from build123d import *

# Parameters (mm, degrees)
F1_DEPTH = 63.5
F2_DEPTH = 25.4
F3_DEPTH = 7.9375
F5_R     = 6.35


with BuildPart() as f1:
    # F0 (on Front) → F1 (new body, symmetric)
    with BuildSketch(Plane.XZ):
        Polygon((-41.275, 9.525), (-41.275, -9.525), (41.275, -9.525), (41.275, 9.525), (23.3043469489, 9.525), align=None)
    extrude(amount=F1_DEPTH, both=True)

    # F0 (on Front) → F2 (join, symmetric)
    with BuildSketch(Plane.XZ):
        with BuildLine():
            Line((23.3043469489, 9.525), (41.275, 9.525))
            Line((41.275, 9.525), (41.275, 32.9785965501))
            ThreePointArc((41.275, 32.9785965501), (47.109768429, 45.2753186743), (60.325, 48.5328564168))
            Line((60.325, 48.5328564168), (60.325, 66.675))
            ThreePointArc((60.325, 66.675), (34.3676792005, 58.0084605019), (23.3043469489, 32.9785965501))
            Line((23.3043469489, 32.9785965501), (23.3043469489, 9.525))
        make_face()
        with BuildLine():
            ThreePointArc((76.3579214275, 60.8458530511), (68.7147538428, 64.787159847), (60.325, 66.675))
            Line((60.325, 66.675), (60.325, 48.5328564168))
            ThreePointArc((60.325, 48.5328564168), (65.4413001724, 46.5163203784), (69.5626091196, 42.8752))
            Line((69.5626091196, 42.8752), (89.6713504766, 42.8752))
            Line((89.6713504766, 42.8752), (89.6713504766, 60.8458530511))
            Line((89.6713504766, 60.8458530511), (76.3579214275, 60.8458530511))
        make_face()
    extrude(amount=F2_DEPTH, both=True)

    # F0 (on Front) → F3 (join, symmetric)
    with BuildSketch(Plane.XZ):
        with BuildLine():
            add(Edge.make_bspline(
                [(-41.275, 9.525), (-31.5447561443, 45.2147647738), (19.8492854834, 73.3103826642), (60.325, 66.675)],
                knots=[0, 0, 0, 0, 116.5705044169, 116.5705044169, 116.5705044169, 116.5705044169], degree=3))
            Line((-41.275, 9.525), (23.3043469489, 9.525))
            Line((23.3043469489, 9.525), (23.3043469489, 32.9785965501))
            ThreePointArc((23.3043469489, 32.9785965501), (34.3676792005, 58.0084605019), (60.325, 66.675))
        make_face()
    extrude(amount=F3_DEPTH, both=True)

    # F0 (on Front) → F4 (revolve)
    with BuildSketch(Plane.XZ):
        Polygon((111.125, 66.675), (89.6713504766, 66.675), (89.6713504766, 60.8458530511), (89.6713504766, 42.8752), (89.6713504766, 38.1), (111.125, 38.1), align=None)
    revolve(axis=Axis((89.6713504766, 0, 52.3875), (0, 0, 1)))

    # F5
    f5_edges = [f1.edges().sort_by_distance(p)[0] for p in [
        (-41.275, -63.5, 0),
        (41.275, -63.5, 0),
        (-41.275, 63.5, 0),
        (41.275, 63.5, 0),
    ]]
    fillet(f5_edges, radius=F5_R)


solid = f1.part
Source: CAD feature listing. Evaluate the final solid. Frame: model axes, mm. A direction names the side the tool comes from. Coordinates: 2 decimals unless noted, no trailing zeros. Order: outer loops, then holes, each group sorted by start corner. A loop starts at its lowest first (then second) coordinate and runs counter-clockwise, first axis right, second up. Notation, with made-up numbers: M 44,80 L 84,80 A33 cw 84,111 Z; hole C 44.25,38 d8. An arc over 180 degrees is marked long. Write each question's results on one line, items separated by ' | '. Start each with the question number.
Item 1: Set-up query: faces 1 (the face through (23.304, 17, 21)), 2 (the face through (77, 20, 42.875)), 3 (the face through (49, -25.4, 51)). Return all of +Z, -Z, +X, -X, +Y, -Y with unobstructed straight access to the full face (end or side cutting, diameter ignored); none if empty.
Item 2: Cut plane A-A (y = 41.5). Return loops of the section in (x, z) (3 decimals).
Item 3: First-contact query: pin 1 Ø12 at (x, z) = (91.5, 47) entering from -Y; pin 2 Ø13 at (y, z) = (-10, 18.5) entering from +X (3 decimals); pin 3 Ø19.5 at (x, y) = (82, -20.5) entering from -Z; pin 4 Ø17 at (x, z) = (58, 36.5) entering from -Y. Flat tips, straight axial feed; report the tip coordinate or a pass-through.
Item 4: Draft query along X for faces 4 (the face through (110.134, 6.444, 52.588)), 5 (the face through (89.671, -23, 52)), 6 (the face through (89, 0, 66.675)). Return one class per face: pulls with the +X half, pulls with the -X half, needs draft (parallel to the pull), parting line crosses it, or undercut.
Item 5: Line query: probe 1 along Z at (x, y) = (-13.5, 39) (3 decimals); probe 2 along Y at (x, z) = (34.5, 23); probe 3 along Y at (x, z) = (15, 53.5). Output: solid intervals per line, ascending.
Checked values:
1) face 1: +Z, -X, +Y | face 2: -Z, +Y | face 3: +Z, +X, -X, -Y
2) outline: M -41.275,-9.525 L 41.275,-9.525 L 41.275,9.525 L -41.275,9.525 Z
3) pin 1: stops at y = -25.4 | pin 2: stops at x = 41.275 | pin 3: stops at z = 38.1 | pin 4: passes through
4) face 4: undercut | face 5: pulls with the +X half | face 6: needs draft
5) probe 1: z = -9.525 to 9.525 | probe 2: y = -25.4 to 25.4 | probe 3: y = -7.94 to 7.94
